from build123d import *
from build123d.topology import SkipClean

# Parameters (mm, degrees)
ESQUISSE1_W              = 22.3
ESQUISSE1_H              = 43
ESQUISSE1_R              = 2.45
BOSS_EXTRU_1_DEPTH       = 5
BOSS_EXTRU_2_START       = -2.47
ESQUISSE2_R              = 2.45
ESQUISSE2_R_2            = 0.7
BOSS_EXTRU_2_DEPTH       = 2.47
ESQUISSE3_W              = 4
ESQUISSE3_H              = 5
ESQUISSE3_W_2            = 3.94
BOSS_EXTRU_3_DEPTH       = 12.3
ESQUISSE4_R              = 0.7
ENL_V_MAT_EXTRU_1_DEPTH  = 52.435201954
BOSS_EXTRU_4_DEPTH       = 1
ESQUISSE6_W              = 10.7
ESQUISSE6_H              = 12.3
BOSS_EXTRU_5_DEPTH       = 1
ESQUISSE7_R              = 0.7
BOSS_EXTRU_6_DEPTH       = 4
BOSS_EXTRU_7_DEPTH       = 2
BOSS_EXTRU_7_DEPTH_BACK  = 5
ESQUISSE10_R             = 18.258884917
ESQUISSE10_R_2           = 10.815915506
ESQUISSE11_R             = 25
ESQUISSE11_R_2           = 18.258884917
ENL_V_MAT_EXTRU_4_DEPTH  = 3
ESQUISSE13_W             = 11.54
ESQUISSE13_H             = 5
BOSS_EXTRU_14_DEPTH      = 12.3
BOSS_EXTRU_15_DEPTH      = 12.3
BOSS_EXTRU_19_DEPTH      = 12.3
BOSS_EXTRU_19_DEPTH_BACK = 1
ESQUISSE16_R             = 0.9
ENL_V_MAT_EXTRU_5_DEPTH  = 54.89147246
ESQUISSE17_R             = 0.9
ENL_V_MAT_EXTRU_6_DEPTH  = 54.891424113


with BuildPart() as part:
    # Esquisse1 → Boss.-Extru.1 (new body)
    with BuildSketch(Plane.XY):
        with Locations((-11.15, -21.5)):
            Rectangle(ESQUISSE1_W, ESQUISSE1_H)
        with Locations((-6.15, -6.15)):
            Circle(ESQUISSE1_R, mode=Mode.SUBTRACT)
    extrude(amount=BOSS_EXTRU_1_DEPTH)

    # Esquisse2 → Boss.-Extru.2 (add)
    with BuildSketch(Plane.XY.offset(5).offset(BOSS_EXTRU_2_START)):
        with Locations((-6.15, -6.15)):
            Circle(ESQUISSE2_R)
        with Locations((-6.15, -6.15)):
            Circle(ESQUISSE2_R_2, mode=Mode.SUBTRACT)
    extrude(amount=BOSS_EXTRU_2_DEPTH)

    # Esquisse3 → Boss.-Extru.3 (add)
    with BuildSketch(Plane.XY.offset(5)):
        with Locations((-20.3, -40.5)):
            Rectangle(ESQUISSE3_W, ESQUISSE3_H)
        with Locations((-13.54, -40.5)):
            Rectangle(ESQUISSE3_W, ESQUISSE3_H)
        with Locations((-20.3, -12.82)):
            Rectangle(ESQUISSE3_W, ESQUISSE3_H)
        with Locations((-13.57, -12.82)):
            Rectangle(ESQUISSE3_W_2, ESQUISSE3_H)
    extrude(amount=BOSS_EXTRU_3_DEPTH)

    # Esquisse4 → Enlèv. mat.-Extru.1 (cut, through all)
    with BuildSketch(Plane.ZY.offset(22.3)):
        with Locations((11.15, -12.82)):
            Circle(ESQUISSE4_R)
        with Locations((11.15, -40.42)):
            Circle(ESQUISSE4_R)
    extrude(amount=-ENL_V_MAT_EXTRU_1_DEPTH, mode=Mode.SUBTRACT)

    # Esquisse5 → Boss.-Extru.4 (add)
    with BuildSketch(Plane.XZ.offset(43)):
        Polygon((-22.3, 17.3), (-11.54, 17.3), (0, 17.3), (0, 5), (0, 0), (-22.3, 0), align=None)
    extrude(amount=BOSS_EXTRU_4_DEPTH)

    # Esquisse6 → Boss.-Extru.5 (add)
    with BuildSketch(Plane(origin=(0, -10.32, 0), x_dir=(1, 0, 0), z_dir=(0, 1, 0))):
        with Locations((-16.95, -11.15)):
            Rectangle(ESQUISSE6_W, ESQUISSE6_H)
    extrude(amount=BOSS_EXTRU_5_DEPTH)

    # Esquisse7 → Boss.-Extru.6 (add)
    with BuildSketch(Plane(origin=(0, 0, 0), x_dir=(0, 0, -1), z_dir=(1, 0, 0))):
        Polygon((-5, -9.32), (0, -9.32), (0, -15.32), (0, -27.62), (0, -44), (-17.3, -44), (-17.3, -9.32), align=None)
        with Locations(Location((-11.15, -21.47, 0), (0, 0, 90))):
            Circle(ESQUISSE7_R, mode=Mode.SUBTRACT)
    extrude(amount=BOSS_EXTRU_6_DEPTH)

    # Esquisse10 → Boss.-Extru.7 (add, two sides: drawn at the far end of the back side and taken through both)
    with BuildSketch(Plane(origin=(0, 0, 0), x_dir=(-1, 0, 0), z_dir=(0, 0, -1)).offset(-BOSS_EXTRU_7_DEPTH_BACK)):
        with Locations((6.15, -6.15)):
            Circle(ESQUISSE10_R)
        with Locations((6.15, -6.15)):
            Circle(ESQUISSE10_R_2, mode=Mode.SUBTRACT)
    extrude(amount=BOSS_EXTRU_7_DEPTH + BOSS_EXTRU_7_DEPTH_BACK)

    # Esquisse11 → Enlèv. mat.-Extru.4 (cut)
    with BuildSketch(Plane(origin=(0, 0, 0), x_dir=(-1, 0, 0), z_dir=(0, 0, -1))):
        with Locations((6.15, -6.15)):
            Circle(ESQUISSE11_R)
        with Locations((6.15, -6.15)):
            Circle(ESQUISSE11_R_2, mode=Mode.SUBTRACT)
    extrude(amount=-ENL_V_MAT_EXTRU_4_DEPTH, mode=Mode.SUBTRACT)

    # Esquisse13 → Boss.-Extru.14 (add, through all)
    with BuildSketch(Plane.XY.offset(5)):
        with Locations((-5.77, -40.5)):
            Rectangle(ESQUISSE13_W, ESQUISSE13_H)
    extrude(amount=BOSS_EXTRU_14_DEPTH)

    # Esquisse14 → Boss.-Extru.15 (add, through all)
    with BuildSketch(Plane.XY.offset(5)):
        with BuildLine():
            Line((-11.6, 11.276542354), (-11.6, -9.32))
            Line((-11.6, -9.32), (-24.131601108, -9.32))
            ThreePointArc((-24.131601108, -9.32), (-21.748537491, 3.340653642), (-11.6, 11.276542354))
        make_face()
    extrude(amount=BOSS_EXTRU_15_DEPTH)

    # Esquisse15 → Boss.-Extru.19 (add, two sides: drawn at the far end of the back side and taken through both)
    with SkipClean():  # the faces are left unmerged after this step: merging them gives an invalid solid
        with BuildSketch(Plane.XY.offset(5).offset(-BOSS_EXTRU_19_DEPTH_BACK)):
            with BuildLine():
                Line((0, 11.041985878), (0, -21.327759335))
                Line((0, -21.327759335), (4, -21.327759335))
                ThreePointArc((4, -21.327759335), (11.971054089, -3.910741832), (0, 11.041985878))
            make_face()
        extrude(amount=BOSS_EXTRU_19_DEPTH + BOSS_EXTRU_19_DEPTH_BACK)

    # Esquisse16 → Enlèv. mat.-Extru.5 (cut, through all)
    with SkipClean():  # the faces are left unmerged after this step: merging them gives an invalid solid
        with BuildSketch(Plane.XY.offset(17.300185)):
            with Locations((9.85, -6.15)):
                Circle(ESQUISSE16_R)
            with Locations((5.163708499, -17.463708499)):
                Circle(ESQUISSE16_R)
            with Locations((-22.15, -6.15)):
                Circle(ESQUISSE16_R)
            with Locations((-17.463708499, 5.163708499)):
                Circle(ESQUISSE16_R)
            with Locations((-6.15, 9.85)):
                Circle(ESQUISSE16_R)
            with Locations((5.163708499, 5.163708499)):
                Circle(ESQUISSE16_R)
        extrude(amount=-ENL_V_MAT_EXTRU_5_DEPTH, mode=Mode.SUBTRACT)

    # Esquisse17 → Enlèv. mat.-Extru.6 (cut, through all)
    with SkipClean():  # the faces are left unmerged after this step: merging them gives an invalid solid
        with BuildSketch(Plane.XY.offset(17.30005)):
            with Locations((-5.77, -40.5)):
                Circle(ESQUISSE17_R)
        extrude(amount=-ENL_V_MAT_EXTRU_6_DEPTH, mode=Mode.SUBTRACT)


solid = part.part
Input: part model. Units: mm. Frame: model coordinates. A direction names the side the tool comes from. Give positions to 0.01 mm unless a question says otherwise; leave off trailing zeros. Order: outer loops, then holes, each group sorted by start corner. A loop starts at its lowest first (then second) coordinate and runs counter-clockwise, first axis right, second up. Notation, with made-up numbers: M -25,87.5 L -17,87.5 A27 ccw -17,117.5 Z; hole C 57.25,-10.5 d6. An arc over 180 degrees is marked long. Answer as a JSON object with one key per item and string values.
1. Ray query, line 1 (Y direction, x = 5.5, z = 14.75); line 2 (X direction, y = -14, z = 16.5); line 3 (Y direction, x = -22.15, z = 12.25). Return the intervals inside material, ascending. Write a range as [from, to].
Result sheet:
{"line 1": "[-20.21, -18.3], [-16.63, 4.33], [6, 7.91]", "line 2": "[-22.3, -18.3], [-15.54, -11.6], [0, 10.34]", "line 3": "[-44, -38], [-15.32, -7.05], [-5.25, 2.65]"}
2. Cut plane D-D, the plane y = -33. Output: boundary loops of the cut face in (x, z).
Result sheet:
{"outline": "M -22.3,0 L 4,0 L 4,17.3 L 0,17.3 L 0,5 L -22.3,5 Z"}
3. Pull-direction query (X, two-part tool) for faces 1 (the flat face through (-11.54, -40, 11)), 2 (the flat face through (4, -33, 9)), 3 (the flat face through (2, -9.32, 2)), 4 (the cylindrical face through (-13.568, -39.726, 11.059)); classes: +X half, -X half, draft (parallel to the pull), parting line (faces both ways), or undercut.
Result sheet:
{"face 1": "-X half", "face 2": "+X half", "face 3": "undercut", "face 4": "draft"}
4. Cut plane C-C, the plane z = 15.5. Output: boundary loops of the cut face in (x, y).
Result sheet:
{"outline": "M -24.13,-9.32 L -22.3,-9.32 L -22.3,-15.32 L -18.3,-15.32 L -18.3,-10.32 L -15.54,-10.32 L -15.54,-15.32 L -11.6,-15.32 L -11.6,11.28 A18.26 ccw Z; M -22.3,-44 L 4,-44 L 4,-21.33 A18.26 ccw 0,11.04 L 0,-38 L -15.54,-38 L -15.54,-43 L -18.3,-43 L -18.3,-38 L -22.3,-38 Z; hole C -22.15,-6.15 d1.8; hole C -17.46,5.16 d1.8; hole C -5.77,-40.5 d1.8; hole C 5.16,-17.46 d1.8; hole C 5.16,5.16 d1.8; hole C 9.85,-6.15 d1.8"}
5. Cut plane A-A, the plane x = -10.5. Output: boundary loops of the cut face in (y, z), and give its area (3 significant figures).
Result sheet:
{"outline": "M -44,0 L -30.77,0 L -30.77,3 L -23.88,3 L -23.88,-2 L -16.05,-2 L -16.05,0 L 0,0 L 0,5 L -38,5 L -38,17.3 L -44,17.3 Z; M 3.75,-2 L 11.58,-2 L 11.58,5 L 3.75,5 Z", "area": "344 mm²"}
6. Reachability of faces 5 (the cylindrical face through (-20.328, -39.726, 11.059)), 6 (the flat face through (-18.3, -42, 11)), 7 (the cylindrical face through (-9.497, -30.925, 1.479)) from +Z, -Z, +X, -X, +Y, -Y: full face, straight path, thin tool, end or side. Return the list, or none.
Result sheet:
{"face 5": "-X", "face 6": "+Z", "face 7": "-Z"}
7. First-contact query: P1, Ø5, axis at y = -11.5, z = 3, coming from the +X side; P2, Ø1.6, axis at x = -13.5, y = 1, coming from the -Z side; P3, Ø1.3, axis at y = -21.47, z = 11.15, coming from the -X side; P4, Ø2, axis at x = -23.5, z = 8.5, coming from the -Y side. Flat tips, straight axial feed; report the tip coordinate or a pass-through.
Result sheet:
{"P1": "x = 11.89", "P2": "z = -2", "P3": "x = 0", "P4": "y = -9.32"}
8. Cut plane B-B, the plane y = -6.15. State how many separate pieces and enclosed holes the cut face has, and give its area (3 significant figures).
Result sheet:
{"separate pieces": "4", "enclosed holes": "0", "area": "415 mm²"}
